CAD build for the part. Positions are in the model's coordinates, mm. Face numbers are marked on the shaded views. A direction names the side the tool comes from. Coordinates: 2 decimals unless noted, no trailing zeros. Loops run counter-clockwise (first coordinate to the right, second up) from the corner with the lowest first, then second, coordinate; pieces in that order, holes last. Notation, with made-up numbers: (11.25, 45.5) -> (15.25, 45.5) arc R17 ccw to (15.25, 60.5) -> close; hole circle Ø6 at (-33, 15.5). An arc over 180 degrees is marked (long way). Write each question's results on one line, items separated by ' | '.
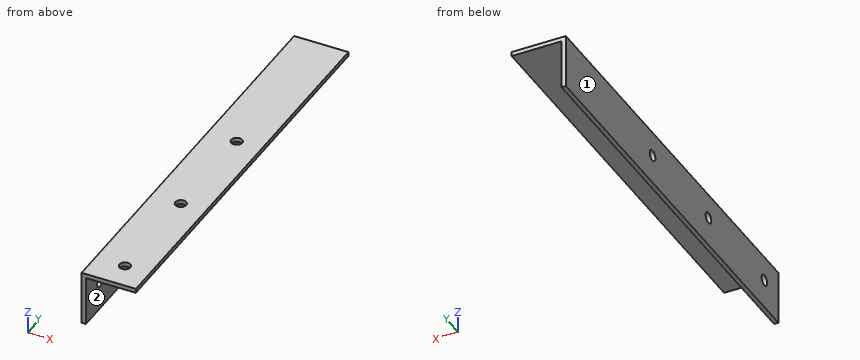
```python
from build123d import *

# Parameters (mm, degrees)
EXTRUDE_1_DEPTH     = 380
SKETCH_2_R          = 5
CUT_EXTRUDE_1_DEPTH = 10
SKETCH_3_R          = 5
CUT_EXTRUDE_2_DEPTH = 10


with BuildPart() as part:
    # Эскиз1 → Вытянуть-Тонкостенный1 (new body)
    with BuildSketch(Plane(origin=(0, 0, 0), x_dir=(1, 0, 0), z_dir=(0, 1, 0))):
        Polygon((0, 50), (0, 0), (50, 0), (50, 4), (4, 4), (4, 50), align=None)
    extrude(amount=EXTRUDE_1_DEPTH)

    # Эскиз2 → Вырез-Вытянуть1 (cut)
    with BuildSketch(Plane.XY):
        with Locations((27, 225)):
            Circle(SKETCH_2_R)
        with Locations((27, 125)):
            Circle(SKETCH_2_R)
        with Locations((27, 25)):
            Circle(SKETCH_2_R)
    extrude(amount=-CUT_EXTRUDE_1_DEPTH, mode=Mode.SUBTRACT)

    # Эскиз3 → Вырез-Вытянуть2 (cut)
    with BuildSketch(Plane.ZY):
        with Locations((-23, 225)):
            Circle(SKETCH_3_R)
        with Locations((-23, 125)):
            Circle(SKETCH_3_R)
        with Locations((-23, 25)):
            Circle(SKETCH_3_R)
    extrude(amount=-CUT_EXTRUDE_2_DEPTH, mode=Mode.SUBTRACT)


solid = part.part
```
Q1. Cut at A-A on y = 25. Write the cut outline in (x, z), and give its area (3 significant figures).
Results are:
outline: (0, -50) -> (4, -50) -> (4, -28) -> (0, -28) -> close; (0, -18) -> (4, -18) -> (4, -4) -> (22, -4) -> (22, 0) -> (0, 0) -> close; (32, -4) -> (50, -4) -> (50, 0) -> (32, 0) -> close | area: 304 mm^2
Q2. Cut at C-C on x = 27. Write the cut outline in (y, z).
Results are:
outline: (0, -4) -> (20, -4) -> (20, 0) -> (0, 0) -> close; (30, -4) -> (120, -4) -> (120, 0) -> (30, 0) -> close; (130, -4) -> (220, -4) -> (220, 0) -> (130, 0) -> close; (230, -4) -> (380, -4) -> (380, 0) -> (230, 0) -> close
Q3. Drop flat-ended pins along their axis: pin 1 (6 mm diameter, centred on y = 327.5, z = -31.5, fed in from +X); pin 2 (4 mm diameter, centred on x = 8.5, y = 255.5, fed in from -Z). Give the stop position or say it passes through.
Results are:
pin 1: x = 4 | pin 2: z = -4
Q4. Cut at D-D on y = 64. Write the cut outline in (x, z).
Results are:
outline: (0, -50) -> (4, -50) -> (4, -4) -> (50, -4) -> (50, 0) -> (0, 0) -> close
Q5. Wall check: L1, parallel to Y at x = 27, z = -1.2; L2, parallel to X at y = 213.5, z = -46.5; L3, parallel to Z at x = 26, y = 257. Give the ranges that are in metal, low to high. Write a range as from..to.
Results are:
L1: 0..20, 30..120, 130..220, 230..380 | L2: 0..4 | L3: -4..0
Q6. Which spindle directions (+Z, -Z, +X, -X, +Y, -Y) get a long thin tool onto all of the face, cutting with end or side? Do the marked faces 1 and 2. Say none if no direction does.
Results are:
face 1: +Z, -Z, -X, +Y, -Y | face 2: -Z, +X, +Y, -Y
Q7. Cut at B-B on z = -23. Write the cut outline in (x, y), and give its area (3 significant figures).
Results are:
outline: (0, 0) -> (4, 0) -> (4, 20) -> (0, 20) -> close; (0, 30) -> (4, 30) -> (4, 120) -> (0, 120) -> close; (0, 130) -> (4, 130) -> (4, 220) -> (0, 220) -> close; (0, 230) -> (4, 230) -> (4, 380) -> (0, 380) -> close | area: 1,400 mm^2
